Can you work these out from the drawing? Everything is in mm from the part's minimum corner. Round coordinates to 2 decimals unless told otherwise and drop trailing zeros. Loops run counter-clockwise (first coordinate to the right, second up) from the corner with the lowest first, then second, coordinate; pieces in that order, holes last. Notation, with made-up numbers: (4, 58) -> (19, 58) arc R25 cw to (19, 82) -> close; hole circle Ø9 at (71.25, 47.5). An arc over 180 degrees is marked (long way). One line per item, written item: value.
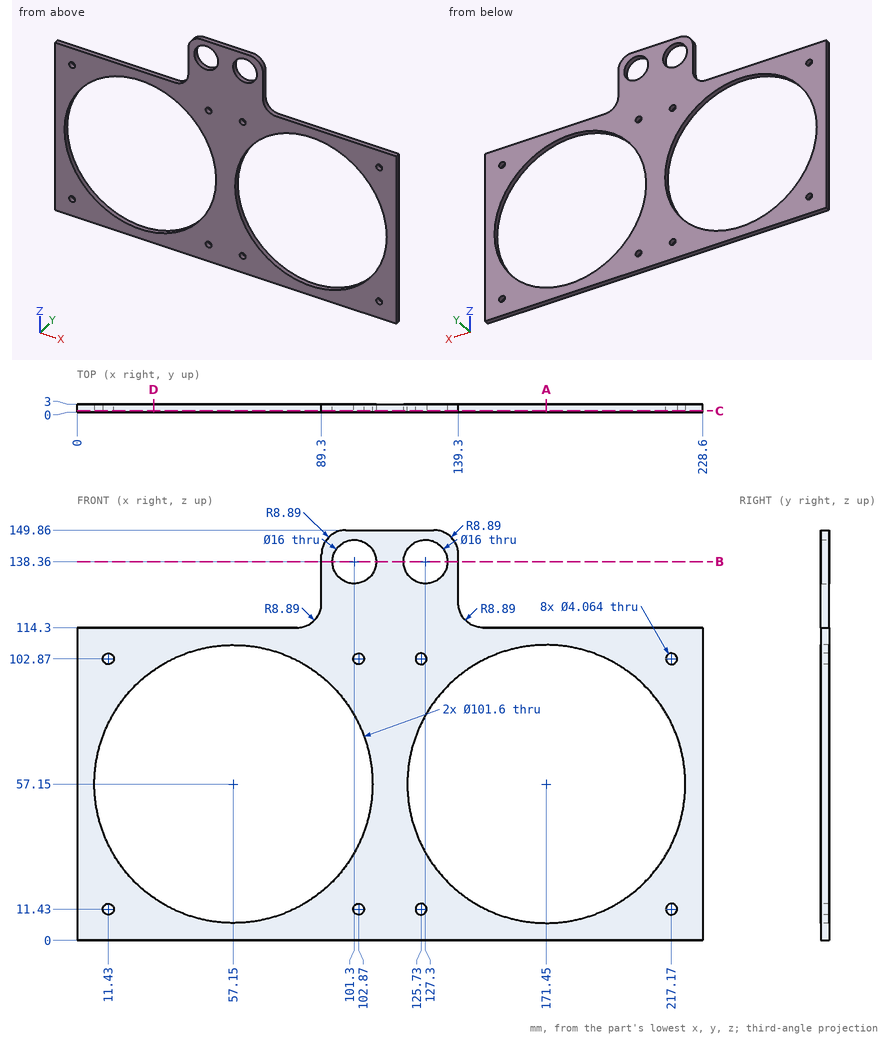
Item 1: I need wall thicknesses on line 1 (X direction, y = 2.55, z = 83); line 2 (X direction, y = 1.25, z = 138.36); line 3 (Z direction, x = 170, y = 0.4). Which ranges of each line are inside material? Lowest first, please. Write a range as from..to.
Output:
line 1: x = 0..13.42, 100.88..127.72, 215.18..228.6
line 2: x = 89.3..93.3, 109.3..119.3, 135.3..139.3
line 3: z = 0..6.37, 107.93..114.3
Item 2: Will these pins go through, and if not, where does the flat tip stop? pin 1 Ø14.5 at (x, z) = (127.3, 138.36) entering from +Y; pin 2 Ø1.5 at (x, y) = (196.5, 1.5) entering from +Z.
Output:
pin 1: passes through
pin 2: stops at z = 114.3
Item 3: If we section it at D-D on x = 28: List the corners of the cut face in (y, z) for me.
Output:
outline: (0, 0) -> (3, 0) -> (3, 15.55) -> (0, 15.55) -> close; (0, 98.75) -> (3, 98.75) -> (3, 114.3) -> (0, 114.3) -> close
Item 4: If we section it at C-C on y = 0.5: Count the separate pieces of the cut face and the enclosed holes in it, plus the area to 3 significant figures.
Output:
separate pieces: 1
enclosed holes: 12
area: 11,200 mm²
Item 5: If we section it at A-A on x = 171.45: List the corners of the cut face in (y, z) for me.
Output:
outline: (0, 0) -> (3, 0) -> (3, 6.35) -> (0, 6.35) -> close; (0, 107.95) -> (3, 107.95) -> (3, 114.3) -> (0, 114.3) -> close
Item 6: If we section it at B-B on z = 138.36: List the corners of the cut face in (x, y) for me.
Output:
outline: (89.3, 0) -> (93.3, 0) -> (93.3, 3) -> (89.3, 3) -> close; (109.3, 0) -> (119.3, 0) -> (119.3, 3) -> (109.3, 3) -> close; (135.3, 0) -> (139.3, 0) -> (139.3, 3) -> (135.3, 3) -> close
